from build123d import *

# Parameters (mm, degrees)
ESQUISSE1_R        = 2.498275285
BOSS_EXTRU_1_DEPTH = 5


with BuildPart() as part:
    # Esquisse1 → Boss.-Extru.1 (new body)
    with BuildSketch(Plane.XY):
        with BuildLine():
            Line((-35, 37.471042471), (35, 37.471042471))
            Line((35, 37.471042471), (35, 42.471042471))
            Line((35, 42.471042471), (70, 42.471042471))
            Line((70, 42.471042471), (70, 37.471042471))
            Line((70, 37.471042471), (95, 37.471042471))
            Line((95, 37.471042471), (95, 42.472767186))
            Line((95, 42.472767186), (100, 42.472767186))
            Line((100, 42.472767186), (100, 37.471042471))
            Line((100, 37.471042471), (100, 27.471042471))
            Line((100, 27.471042471), (95, 27.471042471))
            Line((95, 27.471042471), (95, 7.471042471))
            Line((95, 7.471042471), (100, 7.471042471))
            Line((100, 7.471042471), (100, -2.528957529))
            ThreePointArc((100, -2.528957529), (105, -7.528957529), (100, -12.528957529))
            Line((100, -12.528957529), (100, -22.528957529))
            Line((100, -22.528957529), (95, -22.528957529))
            Line((95, -22.528957529), (95, -42.528957529))
            Line((95, -42.528957529), (100, -42.528957529))
            Line((100, -42.528957529), (100, -52.528957529))
            Line((100, -52.528957529), (100, -57.527232814))
            Line((100, -57.527232814), (95, -57.527232814))
            Line((95, -57.527232814), (95, -52.528957529))
            Line((95, -52.528957529), (70, -52.528957529))
            Line((70, -52.528957529), (70, -57.528957529))
            Line((70, -57.528957529), (35, -57.528957529))
            Line((35, -57.528957529), (35, -52.528957529))
            Line((35, -52.528957529), (-35, -52.528957529))
            Line((-35, -52.528957529), (-35, -57.528957529))
            Line((-35, -57.528957529), (-70, -57.528957529))
            Line((-70, -57.528957529), (-70, -52.528957529))
            Line((-70, -52.528957529), (-95, -52.528957529))
            Line((-95, -52.528957529), (-95, -57.528957529))
            Line((-95, -57.528957529), (-100, -57.528957529))
            Line((-100, -57.528957529), (-100, -52.528957529))
            Line((-100, -52.528957529), (-100, -42.528957529))
            Line((-100, -42.528957529), (-95, -42.528957529))
            Line((-95, -42.528957529), (-95, -22.528957529))
            Line((-95, -22.528957529), (-100, -22.528957529))
            Line((-100, -22.528957529), (-100, -12.528957529))
            ThreePointArc((-100, -12.528957529), (-105, -7.528957529), (-100, -2.528957529))
            Line((-100, -2.528957529), (-100, 7.471042471))
            Line((-100, 7.471042471), (-95, 7.471042471))
            Line((-95, 7.471042471), (-95, 27.471042471))
            Line((-95, 27.471042471), (-100, 27.471042471))
            Line((-100, 27.471042471), (-100, 37.471042471))
            Line((-100, 37.471042471), (-100, 42.471042471))
            Line((-100, 42.471042471), (-95, 42.471042471))
            Line((-95, 42.471042471), (-95, 37.471042471))
            Line((-95, 37.471042471), (-70, 37.471042471))
            Line((-70, 37.471042471), (-70, 42.471042471))
            Line((-70, 42.471042471), (-35, 42.471042471))
            Line((-35, 42.471042471), (-35, 37.471042471))
        make_face()
        with Locations((100, -7.528957529)):
            Circle(ESQUISSE1_R, mode=Mode.SUBTRACT)
        with Locations(Location((-100, -7.528957529, 0), (0, 0, 180))):
            Circle(ESQUISSE1_R, mode=Mode.SUBTRACT)
    extrude(amount=BOSS_EXTRU_1_DEPTH)


solid = part.part
Can you work these out from the model? Positions are in its coordinate system, mm. A direction names the side the tool comes from. Coordinates: 2 decimals unless noted, no trailing zeros. Write each loop counter-clockwise with the first axis right and the second up, starting at its lowest first coordinate (ties: lowest second). Pieces come first, ordered by that corner, then holes. Notation, with made-up numbers: (81, -3) -> (115, -3) arc R8 cw to (115, 8) -> close; hole circle Ø11 at (42.25, 80.5). An arc over 180 degrees is marked (long way). Write each question's results on one line, items separated by ' | '. Start each with the question number.
Q1. Imagine slicing it at A-A (y = -39). Write out the boundary of the cut face in (x, z), then the cut area to 3 significant figures.
Q2. On a 3-axis mill with a long thin cutter (end or side, diameter ignored), from which of +Z, -Z, +X, -X, +Y, -Y can I reach the whole of each face in a straight line? I mean faces 5 (the face through (-95, 17, 2)), 6 (the face through (100, -50, 2)), 7 (the face through (0, -52.529, 2)). Say none if no direction works.
Q3. We'd pull the mould along X, two halves only. Please class faces 1 (the face through (97, 7.471, 2)), 2 (the face through (35, 40, 2)), 3 (the face through (-100, 35, 2)), 4 (the face through (-95, -55, 2)): +X half, -X half, draft (parallel to the pull), parting line (faces both ways), or undercut.
Q4. Imagine slicing it at B-B (x = -78). Write out the boundary of the cut face in (y, z).
Q5. Imagine slicing it at C-C (z = 3.25). State how many separate pieces and enclosed holes the cut face has, then the cut area to 3 significant figures.
Q6. I'm going to push flat-ended pins straight in: pin 1 (2.5 mm diameter, centred on y = 1.5, z = 3.5, fed in from +X); pin 2 (2.5 mm diameter, centred on x = 7.5, z = 1.5, fed in from +Y); pin 3 (1.5 mm diameter, centred on x = 8.5, z = 3.5, fed in from -Y); pin 4 (4.5 mm diameter, centred on x = -100, y = -7.53, fed in from -Z). Where does each tip first touch, or does it pass through?
Q7. If I drill on probe 1 along X at (y, z) = (-6, 2.8); probe 2 along Y at (x, z) = (1, 4.7); probe 3 along Y at (x, z) = (42, 4.4), over which ranges is the centre line in solid material (lowest first)?
Taken from the geometry:
1) outline: (-95, 0) -> (95, 0) -> (95, 5) -> (-95, 5) -> close | area: 950 mm^2
2) face 5: +Z, -Z, -X | face 6: +Z, -Z, +X, -Y | face 7: +Z, -Z, -Y
3) face 1: draft | face 2: undercut | face 3: -X half | face 4: undercut
4) outline: (-52.53, 0) -> (37.47, 0) -> (37.47, 5) -> (-52.53, 5) -> close
5) separate pieces: 1 | enclosed holes: 2 | area: 18,400 mm^2
6) pin 1: stops at x = 100 | pin 2: stops at y = 37.47 | pin 3: stops at y = -52.53 | pin 4: passes through
7) probe 1: x = -104.76 to -101.98, -98.02 to 98.02, 101.98 to 104.76 | probe 2: y = -52.53 to 37.47 | probe 3: y = -57.53 to 42.47
